Print and shaded views of the part. All mm, measured from the part's lowest x, y and z. A direction names the side the tool comes from. Round coordinates to 2 decimals unless told otherwise and drop trailing zeros. Loops run counter-clockwise (first coordinate to the right, second up) from the corner with the lowest first, then second, coordinate; pieces in that order, holes last. Notation, with made-up numbers: (-13.75, 34) - (-9.75, 34) arc R22 ccw to (-9.75, 65) - close; hole circle Ø5 at (-4.75, 10). An arc over 180 degrees is marked (long way). Answer as a JSON object with one key per item and string values.
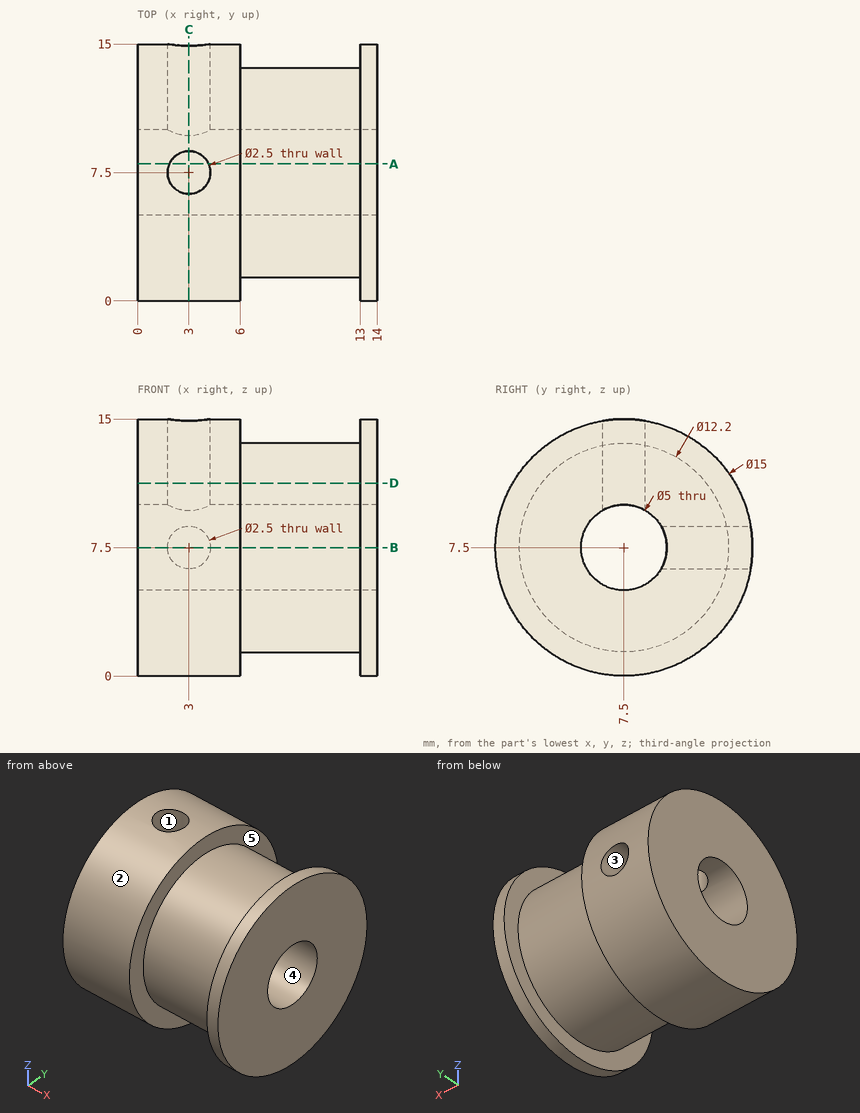
1) Slice it at B-B on z = 7.5. List the corners of the cut face in (x, y), then the cut area to 3 significant figures.
Values follow:
{"outline": "(0, 0) - (6, 0) - (6, 1.4) - (13, 1.4) - (13, 0) - (14, 0) - (14, 5) - (0, 5) - close; (0, 10) - (1.75, 10) - (1.75, 15) - (0, 15) - close; (4.25, 10) - (14, 10) - (14, 15) - (13, 15) - (13, 13.6) - (6, 13.6) - (6, 15) - (4.25, 15) - close", "area": "108 mm²"}
2) Two-plate mould, pull along Z, no slides. Class the marked faces 1, 2 and 3: pulls with the +Z half, pulls with the -Z half, needs draft (parallel to the pull), parting line crosses it, or undercut.
Values follow:
{"face 1": "needs draft", "face 2": "parting line crosses it", "face 3": "undercut"}
3) Slice it at C-C on x = 3. List the corners of the cut face in (y, z).
Values follow:
{"outline": "(6.25, 9.67) - (6.25, 14.9) arc R7.5 ccw (long way) to (14.9, 6.25) - (9.67, 6.25) arc R2.5 cw (long way) to start; (8.75, 9.67) arc R2.5 cw to (9.67, 8.75) - (14.9, 8.75) arc R7.5 ccw to (8.75, 14.9) - close"}
4) Drop flat-ended pins along their axis: P1, Ø1.5, axis at x = 2.5, z = 6.5, coming from the -Y side; P2, Ø1.5, axis at x = 9.5, z = 13.5, coming from the -Y side; P3, Ø1.5, axis at x = 7.5, z = 6, coming from the +Y side; P4, Ø8, axis at x = 12, y = 6.5, coming from the -Z side. Give the stop position or say it passes through.
Values follow:
{"P1": "y = 0", "P2": "y = 4.39", "P3": "y = 13.55", "P4": "z = 0"}
5) Tool access for the marked faces 4 and 5: list every direction of +Z, -Z, +X, -X, +Y, -Y with a clear straight run to the whole face (end or side of a thin tool).
Values follow:
{"face 4": "+X, -X", "face 5": "none"}
6) Probe probe 1 along X at (y, z) = (7.25, 14.25); probe 2 along X at (y, z) = (1.5, 4.5); probe 3 along Z at (x, y) = (4, 7.5). List the from-to ranges inside material, lowest first.
Values follow:
{"probe 1": "0 to 1.78, 4.22 to 6, 13 to 14", "probe 2": "0 to 6, 13 to 14", "probe 3": "0 to 5"}
7) Slice it at D-D on z = 11.25. List the corners of the cut face in (x, y), then the cut area to 3 significant figures.
Values follow:
{"outline": "(0, 1) - (6, 1) - (6, 2.69) - (13, 2.69) - (13, 1) - (14, 1) - (14, 14) - (13, 14) - (13, 12.31) - (6, 12.31) - (6, 14) - (0, 14) - close; hole circle Ø2.5 at (3, 7.5)", "area": "153 mm²"}
8) Slice it at A-A on y = 8. List the corners of the cut face in (x, z).
Values follow:
{"outline": "(0, 0.02) - (6, 0.02) - (6, 1.42) - (13, 1.42) - (13, 0.02) - (14, 0.02) - (14, 5.05) - (0, 5.05) - close; (0, 9.95) - (1.85, 9.95) - (1.85, 14.98) - (0, 14.98) - close; (4.15, 9.95) - (14, 9.95) - (14, 14.98) - (13, 14.98) - (13, 13.58) - (6, 13.58) - (6, 14.98) - (4.15, 14.98) - close"}
